Input: part model. Units: mm. Frame: model coordinates. A direction names the side the tool comes from. Round coordinates to 2 decimals unless told otherwise and drop trailing zeros. Order: outer loops, then holes, each group sorted by start corner. A loop starts at its lowest first (then second) coordinate and runs counter-clockwise, first axis right, second up. Notation, with made-up numbers: (29.5, 48.5) -> (73.5, 48.5) arc R10 ccw to (73.5, 67.5) -> close; hole circle Ø2 at (83, 20.5). An arc over 180 degrees is marked (long way). Answer as CSV lines item,"result". Start each with the question number.
1) Mould query, pull axis X, two halves, no side actions, for faces 1 (the face through (-1, 0, -127)), 2 (the face through (-55.88, 0, 2)), 3 (the face through (-40.44, 0.178, -78.346)). Classes: +X half, -X half, draft (parallel to the pull), parting line (faces both ways), or undercut.
2) Section query B-B, the plane x = 0. Output: boundary loops of the cut face in (y, z) (3 decimals), and give its area (3 significant figures).
3) Line query: L1, parallel to X at y = 6.25, z = -76.2 (3 decimals); L2, parallel to Z at x = -7.5, y = 6.5; L3, parallel to Z at x = 38.1, y = 6.75 (3 decimals). Output: solid intervals per line, ascending.
4) Section query C-C, the plane y = 2.5. Output: boundary loops of the cut face in (x, z) (3 decimals).
5) Access query for faces 4 (the face through (-38, 12.7, -2)), 5 (the face through (0, 0, 31.75)). Directions: +Z, -Z, +X, -X, +Y, -Y. A direction counts if a zero-diameter tool reaches every point of the face in a straight line with its end or side. Return the directions, or none.
6) Section query D-D, the plane z = -76.2. Output: boundary loops of the cut face in (x, y) (3 decimals), and give its area (3 significant figures).
7) First-contact query: P1, Ø10, axis at x = -38.1, z = -76.2, coming from the +Y side. Flat tip, straight axial feed; report the tip coordinate or a pass-through.
8) Section query A-A, the plane z = 76.2. Output: boundary loops of the cut face in (x, y) (3 decimals).
```python
from build123d import *

# Parameters (mm, degrees)
SKETCH1_W           = 111.76
SKETCH1_H           = 254
BOSS_EXTRUDE1_DEPTH = 12.7
SKETCH2_W           = 63.5
SKETCH2_H           = 63.5
CUT_EXTRUDE1_DEPTH  = 25.4
CUT_EXTRUDE2_REACH  = 27.4
SKETCH3_R           = 3.175


with BuildPart() as part:
    # Sketch1 → Boss-Extrude1 (new body, symmetric)
    with BuildSketch(Plane(origin=(0, 0, 0), x_dir=(1, 0, 0), z_dir=(0, 1, 0))):
        Rectangle(SKETCH1_W, SKETCH1_H)
    extrude(amount=BOSS_EXTRUDE1_DEPTH, both=True)

    # Sketch2 → Cut-Extrude1 (cut)
    with BuildSketch(Plane(origin=(0, 12.7, 0), x_dir=(1, 0, 0), z_dir=(0, 1, 0))):
        Rectangle(SKETCH2_W, SKETCH2_H)
    extrude(amount=-CUT_EXTRUDE1_DEPTH, mode=Mode.SUBTRACT)

    # Sketch3 → Cut-Extrude2 (cut, up to next)
    with BuildSketch(Plane(origin=(0, 12.7, 0), x_dir=(1, 0, 0), z_dir=(0, 1, 0)), mode=Mode.PRIVATE) as cut_extrude2_sk1:
        with Locations((0, -76.2)):
            Circle(SKETCH3_R)
    cut_extrude2_tool1 = extrude(cut_extrude2_sk1.sketch, amount=-CUT_EXTRUDE2_REACH, mode=Mode.PRIVATE) & part.part
    add(cut_extrude2_tool1.solids().sort_by_distance((0, 12.7, 76.2))[0], mode=Mode.SUBTRACT)
    # Sketch3 → Cut-Extrude2 (cut, up to next)
    with BuildSketch(Plane(origin=(0, 12.7, 0), x_dir=(1, 0, 0), z_dir=(0, 1, 0)), mode=Mode.PRIVATE) as cut_extrude2_sk2:
        with Locations((38.1, 76.2)):
            Circle(SKETCH3_R)
    cut_extrude2_tool2 = extrude(cut_extrude2_sk2.sketch, amount=-CUT_EXTRUDE2_REACH, mode=Mode.PRIVATE) & part.part
    add(cut_extrude2_tool2.solids().sort_by_distance((38.1, 12.7, -76.2))[0], mode=Mode.SUBTRACT)
    # Sketch3 → Cut-Extrude2 (cut, up to next)
    with BuildSketch(Plane(origin=(0, 12.7, 0), x_dir=(1, 0, 0), z_dir=(0, 1, 0)), mode=Mode.PRIVATE) as cut_extrude2_sk3:
        with Locations((-38.1, 76.2)):
            Circle(SKETCH3_R)
    cut_extrude2_tool3 = extrude(cut_extrude2_sk3.sketch, amount=-CUT_EXTRUDE2_REACH, mode=Mode.PRIVATE) & part.part
    add(cut_extrude2_tool3.solids().sort_by_distance((-38.1, 12.7, -76.2))[0], mode=Mode.SUBTRACT)


solid = part.part
```
Findings:
1,face 1,"draft"
1,face 2,"-X half"
1,face 3,"undercut"
2,outline,"(-12.7, -127) -> (12.7, -127) -> (12.7, -31.75) -> (-12.7, -31.75) -> close; (-12.7, 31.75) -> (12.7, 31.75) -> (12.7, 73.025) -> (-12.7, 73.025) -> close; (-12.7, 79.375) -> (12.7, 79.375) -> (12.7, 127) -> (-12.7, 127) -> close"
2,area,"4,680 mm^2"
3,L1,"x = -55.88 to -41.275, -34.925 to 34.925, 41.275 to 55.88"
3,L2,"z = -127 to -31.75, 31.75 to 127"
3,L3,"z = -127 to -79.375, -73.025 to 127"
4,outline,"(-55.88, -127) -> (55.88, -127) -> (55.88, 127) -> (-55.88, 127) -> close; hole circle Ø6.35 at (-38.1, -76.2); hole (-31.75, -31.75) -> (31.75, -31.75) -> (31.75, 31.75) -> (-31.75, 31.75) -> close; hole circle Ø6.35 at (0, 76.2); hole circle Ø6.35 at (38.1, -76.2)"
5,face 4,"+Z, -Z, +X, -X, +Y"
5,face 5,"+Y, -Y"
6,outline,"(-55.88, -12.7) -> (-41.275, -12.7) -> (-41.275, 12.7) -> (-55.88, 12.7) -> close; (-34.925, -12.7) -> (34.925, -12.7) -> (34.925, 12.7) -> (-34.925, 12.7) -> close; (41.275, -12.7) -> (55.88, -12.7) -> (55.88, 12.7) -> (41.275, 12.7) -> close"
6,area,"2,520 mm^2"
7,P1,"stops at y = 12.7"
8,outline,"(-55.88, -12.7) -> (-3.175, -12.7) -> (-3.175, 12.7) -> (-55.88, 12.7) -> close; (3.175, -12.7) -> (55.88, -12.7) -> (55.88, 12.7) -> (3.175, 12.7) -> close"
